Verification items for the finished model (mm, model axes). Face numbers are marked on the shaded views. A direction names the side the tool comes from. Coordinates: 2 decimals unless noted, no trailing zeros. Loops run counter-clockwise (first coordinate to the right, second up) from the corner with the lowest first, then second, coordinate; pieces in that order, holes last. Notation, with made-up numbers: (37.5, 83.5) - (70.5, 83.5) arc R11 ccw to (70.5, 103.5) - close; hole circle Ø8 at (76, 31.5). An arc over 180 degrees is marked (long way). One line per item, written item: value. Start each with the question number.
(1) Set-up check for the marked faces 1 and 2: record each of +Z, -Z, +X, -X, +Y, -Y from which the full face is reachable in a straight line by a thin tool's end or side.
(2) Gauge pin test, flat ends, axial feed: P1, Ø20, axis at x = 171.5, z = -171, coming from the +Y side; P2, Ø1.5, axis at x = 139, y = 40, coming from the -Z side; P3, Ø6.5, axis at x = 168.21, z = -172.94, coming from the -Y side; P4, Ø11, axis at y = 3.5, z = -166.5, coming from the +X side. Record the tip position at first contact, or that the pin passes through.
(3) Section check A-A (x = 161.5). Record the boundary of the cut face in (y, z).
(4) Thickness scan on probe 1 along X at (y, z) = (5, -161.5); probe 2 along Z at (x, y) = (190, 37). Record the ranges inside material, lowest first. Write a range as [from, to].
(5) Section check C-C (x = 77). Record the boundary of the cut face in (y, z), plus the area to 4 significant figures.
(6) Section check B-B (y = 43.5). Record the boundary of the cut face in (x, z), plus the area to 3 significant figures.
```python
from build123d import *

# Parameters (mm, degrees)
SKETCH_1_W          = 210
SKETCH_1_H          = 157.5
EXTRUDE_1_DEPTH     = 10
SKETCH_2_W          = 210
SKETCH_2_H          = 157.5
EXTRUDE_2_DEPTH     = 40
SKETCH_3_R          = 3.79044749
SKETCH_3_R_2        = 3.951540246
CUT_EXTRUDE_1_DEPTH = 40


with BuildPart() as part:
    # 草图1 → 凸台-拉伸1 (new body)
    with BuildSketch(Plane(origin=(0, 0, 0), x_dir=(1, 0, 0), z_dir=(0, 1, 0))):
        with Locations((105, 78.75)):
            Rectangle(SKETCH_1_W, SKETCH_1_H)
        with BuildLine():
            Line((34.056494748, 172.5), (34.056494748, 157.5))
            Line((34.056494748, 157.5), (59.056494748, 157.5))
            Line((59.056494748, 157.5), (59.056494748, 172.5))
            ThreePointArc((59.056494748, 172.5), (56.12756256, 179.571067812), (49.056494748, 182.5))
            Line((49.056494748, 182.5), (44.056494748, 182.5))
            ThreePointArc((44.056494748, 182.5), (36.985426936, 179.571067812), (34.056494748, 172.5))
        make_face()
        with BuildLine():
            Line((156.491132728, 157.5), (181.491132728, 157.5))
            Line((181.491132728, 157.5), (181.491132728, 172.5))
            ThreePointArc((181.491132728, 172.5), (178.56220054, 179.571067812), (171.491132728, 182.5))
            Line((171.491132728, 182.5), (166.491132728, 182.5))
            ThreePointArc((166.491132728, 182.5), (159.420064916, 179.571067812), (156.491132728, 172.5))
            Line((156.491132728, 172.5), (156.491132728, 157.5))
        make_face()
    extrude(amount=EXTRUDE_1_DEPTH)

    # 草图2 → 凸台-拉伸2 (add)
    with BuildSketch(Plane(origin=(0, 10, 0), x_dir=(1, 0, 0), z_dir=(0, 1, 0))):
        with Locations((105, 78.75)):
            Rectangle(SKETCH_2_W, SKETCH_2_H)
    extrude(amount=EXTRUDE_2_DEPTH)

    # 草图3 → 切除-拉伸1 (cut)
    with BuildSketch(Plane(origin=(0, 10, 0), x_dir=(1, 0, 0), z_dir=(0, 1, 0))):
        with Locations(Location((46.4811838, 172.938422578, 0), (0, 0, 270))):
            Circle(SKETCH_3_R)
        with Locations(Location((168.209255667, 172.938422578, 0), (0, 0, 270))):
            Circle(SKETCH_3_R_2)
    extrude(amount=-CUT_EXTRUDE_1_DEPTH, mode=Mode.SUBTRACT)


solid = part.part
```
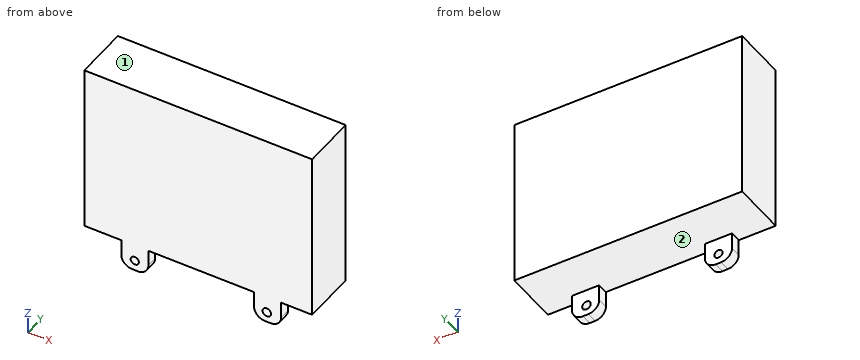
Responses:
1. face 1: +Z, +X, -X, +Y, -Y
1. face 2: -Z, +Y
2. P1: stops at y = 10
2. P2: stops at z = -157.5
2. P3: passes through
2. P4: stops at x = 181.49
3. outline: (0, -181.17) - (10, -181.17) - (10, -157.5) - (50, -157.5) - (50, 0) - (0, 0) - close
4. probe 1: x = [34.06, 59.06], [156.49, 181.49]
4. probe 2: z = [-157.5, 0]
5. outline: (0, -157.5) - (50, -157.5) - (50, 0) - (0, 0) - close
5. area: 7,875 mm²
6. outline: (0, -157.5) - (210, -157.5) - (210, 0) - (0, 0) - close
6. area: 33,100 mm²
